Verification items for this drawing (mm, ordinates from the low corner). Round coordinates to 2 decimals unless told otherwise and drop trailing zeros. Write each loop counter-clockwise with the first axis right and the second up, starting at its lowest first coordinate (ties: lowest second). Pieces come first, ordered by that corner, then holes. Notation, with made-up numbers: (76.25, 45.25) - (89.25, 45.25) arc R28 cw to (89.25, 68.25) - close; hole circle Ø7 at (33, 56.25). An arc over 180 degrees is marked (long way). One line per question, with ' | ' between items. Start each with the question number.
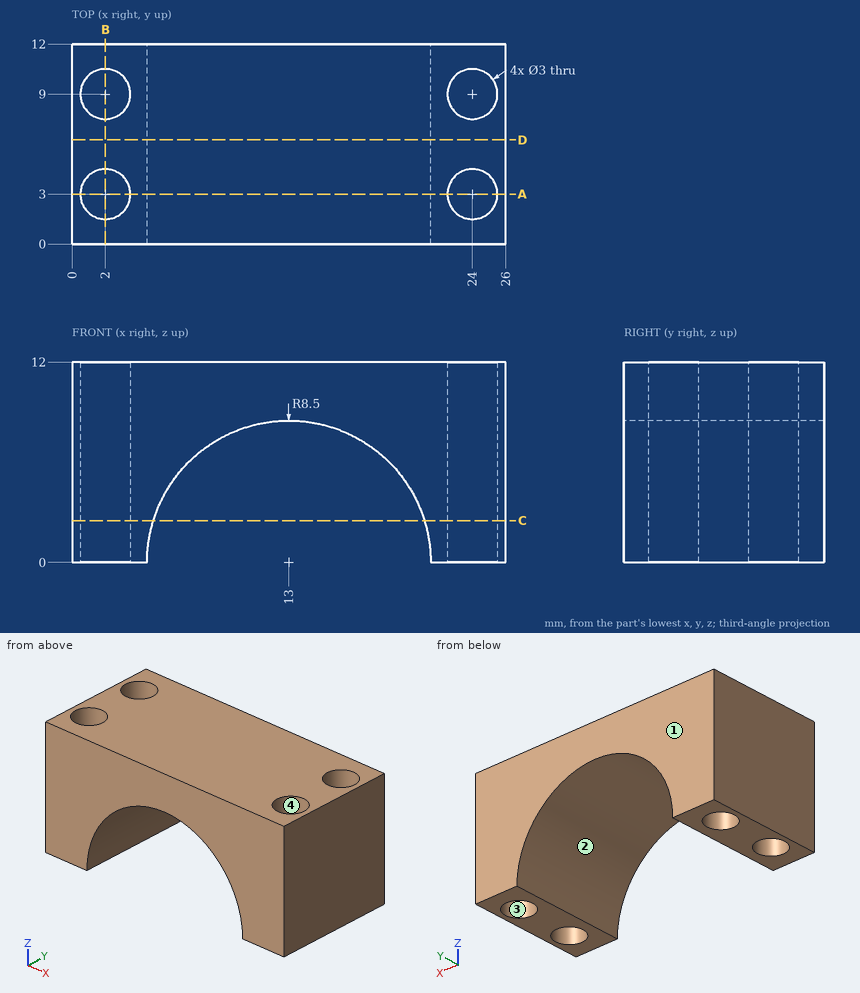
Q1. Section check D-D, the plane y = 6.25. Record the cut outline in (x, z).
Q2. Draft check along Y on the marked faces 1, 2, 3 and 4. Enter one of: pulls with the +Y half, pulls with the -Y half, needs draft (parallel to the pull), parting line crosses it, or undercut.
Q3. Thickness scan on line 1 (Y direction, x = 24, z = 8.5); line 2 (X direction, y = 3.5, z = 6.25) (1 decimal); line 3 (X direction, y = 3.5, z = 1) (1 decimal). Record the ranges inside material, lowest first.
Q4. Section check C-C, the plane z = 2.5. Record the cut outline in (x, y).
Q5. Go/stop test with a flat-tipped pin: P1, Ø5, axis at y = 10.5, z = 4.5, coming from the -X side. Record where the tip stops, or that it passes through.
Q6. Section check A-A, the plane y = 3. Record the cut outline in (x, z).
Q7. Section check B-B, the plane x = 2. Record the cut outline in (y, z).
Result sheet:
1) outline: (0, 0) - (4.5, 0) arc R8.5 cw to (21.5, 0) - (26, 0) - (26, 12) - (0, 12) - close
2) face 1: pulls with the +Y half | face 2: needs draft | face 3: undercut | face 4: undercut
3) line 1: 0 to 1.5, 4.5 to 7.5, 10.5 to 12 | line 2: 0 to 0.6, 3.4 to 7.2, 18.8 to 22.6, 25.4 to 26 | line 3: 0 to 0.6, 3.4 to 4.6, 21.4 to 22.6, 25.4 to 26
4) outline: (0, 0) - (4.88, 0) - (4.88, 12) - (0, 12) - close; (21.12, 0) - (26, 0) - (26, 12) - (21.12, 12) - close; hole circle Ø3 at (2, 3); hole circle Ø3 at (2, 9); hole circle Ø3 at (24, 3); hole circle Ø3 at (24, 9)
5) P1: x = 0
6) outline: (0, 0) - (0.5, 0) - (0.5, 12) - (0, 12) - close; (3.5, 0) - (4.5, 0) arc R8.5 cw to (21.5, 0) - (22.5, 0) - (22.5, 12) - (3.5, 12) - close; (25.5, 0) - (26, 0) - (26, 12) - (25.5, 12) - close
7) outline: (0, 0) - (1.5, 0) - (1.5, 12) - (0, 12) - close; (4.5, 0) - (7.5, 0) - (7.5, 12) - (4.5, 12) - close; (10.5, 0) - (12, 0) - (12, 12) - (10.5, 12) - close
